Geometry check sheet. Reference: the model listing, model coordinates, mm. Give positions to 0.01 mm unless a question says otherwise; leave off trailing zeros. Loops run counter-clockwise (first coordinate to the right, second up) from the corner with the lowest first, then second, coordinate; pieces in that order, holes last. Notation, with made-up numbers: (6, 46.25) -> (55, 46.25) arc R18 cw to (55, 79.25) -> close; hole circle Ø3 at (67.25, -35.75). An arc over 180 degrees is marked (long way). Answer as a JSON object with one key per item and string values.
Autodesk Inventor part; units mm, degrees
ref_plane "YZ Plane" through (0, 0, 0) normal (1, 0, 0) x (0, 1, 0)
ref_plane "XZ Plane" through (0, 0, 0) normal (0, 1, 0) x (-1, 0, 0)
ref_plane "XY Plane" through (0, 0, 0) normal (0, 0, 1) x (1, 0, 0)
sketch "Sketch1" plane through (0, 0, 0) normal (0, 0, 1) x (1, 0, 0)
  circle A0 centre (0, 0) radius 6.35
  dimension "d0" = 12.7
extrude "Extrusion1" add sketch "Sketch1" along normal blind 26.9875 and the other way blind 66.675
sketch "Sketch2" plane through (0, 0, 0) normal (0, 0, 1) x (1, 0, 0)
  circle A0 centre (0, 0) radius 7.1437
  dimension "d5" = 14.2875
extrude "Extrusion2" add sketch "Sketch2" along normal blind 1.5875
chamfer "Chamfer1" distance 4.7625 angle 15 1 edges at (-6.35, 0, -66.675) measured on face at (6.3294, -0.511, -44.45)
chamfer "Chamfer2" distance 1.5875 angle 45 1 edges at (-6.35, 0, 26.9875)
sketch "Sketch3" plane through (0, 0, 0) normal (1, 0, 0) x (0, 1, 0)
  line L0 (0, -53.1813) -> (8.128, -53.1813)
  arc A0 (8.128, -53.1813) -> (5.7468, -50.8) centre (5.7468, -53.1813) ccw
  line L1 (5.7468, -50.8) -> (0, -50.8)
  line L2 (0, -50.8) -> (0, -53.1813)
  point P0 (0, 0)
  dimension "d14" = 4.7625
  dimension "d15" = 50.8
  dimension "d16" = 8.128
revolve "Revolution1" add sketch "Sketch3" angle 360 about axis through (0, 0, -53.1813) along (0, 1, 0)
sketch "Sketch4" plane through (0, 0, 0) normal (1, 0, 0) x (0, 1, 0)
  circle A0 centre (0, 34.925) radius 15.875
  point P0 (0, 0)
  dimension "d18" = 31.75
  dimension "d19" = 34.925
sketch "Sketch5" plane through (0, 0, 0) normal (0, 1, 0) x (-1, 0, 0)
  line L0 (0, 50.8) -> (0, 19.05) construction
  circle A0 centre (0, 50.8) radius 0.7937
  point P0 (0, 0)
  dimension "d20" = 1.5875
sweep "Sweep1" add profiles "Sketch5" path "Sketch4"
properties part number "Quick release pin" material "Stainless Steel"
1) Draft check along Y on faces 1 (the face through (-1.15, -5.17, -65.85)), 2 (the face through (0, 0, 26.988)), 3 (the face through (-6, -3, 1.588)). Enter one of: pulls with the +Y half, pulls with the -Y half, needs draft (parallel to the pull), parting line crosses it, or undercut.
Geometry check:
{"face 1": "parting line crosses it", "face 2": "undercut", "face 3": "needs draft"}
2) Section check B-B on z = -39. Record the cut outline in (x, y), plus the area to 3 significant figures.
Geometry check:
{"outline": "circle Ø12.7 at (0, 0)", "area": "127 mm2"}
3) Material ranges on line 1 along Z through (x, y) = (-3, 0.5) (1 decimal); line 2 along Z through (x, y) = (1.5, 6.5); line 3 along Y through (x, z) = (-0.5, 34), recorded low to high. Write a range as from..to.
Geometry check:
{"line 1": "z = -66.7..27", "line 2": "z = -54.87..-51.49, 0..1.59", "line 3": "y = -16.47..-15.23, 15.23..16.47"}
4) Depth check by flat-ended pin: P1, Ø5, axis at y = 7.5, z = -46.5, coming from the -X side; P2, Ø1.5, axis at x = 2, z = -30, coming from the +Y side; P3, Ø4.5, axis at x = -3.5, y = 2, coming from the +Z side. Enter the tip coordinate at first touch or a pass-through.
Geometry check:
{"P1": "stops at x = -3.91", "P2": "stops at y = 6.23", "P3": "stops at z = 26.99"}
